Check sheet for the modelled part. Datum: model origin and axes. Units: mm. A direction names the side the tool comes from. Give positions to 0.01 mm unless a question says otherwise; leave off trailing zeros. Write each loop counter-clockwise with the first axis right and the second up, starting at its lowest first coordinate (ties: lowest second). Pieces come first, ordered by that corner, then holes. Notation, with made-up numbers: M -11.75,-35 L 6.25,-35 A28 ccw 6.25,4 Z; hole C 66,55 d1. An arc over 180 degrees is marked long. Write item = value, one per line. Start each with the question number.
1) Cross-section at A-A, the plane x = 24.5. Record the cut outline in (y, z), plus the area to 3 significant figures.
2) Go/stop test with flat-tipped pins: pin 1 (8 mm diameter, centred on x = -19.5, y = 4, fed in from -Z); pin 2 (8.5 mm diameter, centred on x = 1.5, z = 253.5, fed in from +Y); pin 3 (4 mm diameter, centred on x = 11.5, y = 13.5, fed in from +Z). Record where each tip stops, or that it passes through.
3) Scan lines: line 1 along Z through (x, y) = (-3, 17.5); line 2 along Y through (x, z) = (-28.5, 328.5); line 3 along Z through (x, y) = (-11, 3.25). Record each from-to range of solid material in increasing order. Write a range as [from, to].
4) Mould release check, pull along X, two halves, no side actions. Record for faces 4 (the cylindrical face through (-3.9, 3.4, 198.1)), 5 (the flat face through (-31.75, 7, 95)), 6 (the flat face through (0, 0, 174)): released by +X, released by -X, zero draft, split by the parting line, or undercut.
5) Cross-section at B-B, the plane y = 14.5. Record the cut outline in (x, z), plus the area to 3 significant figures.
6) Access from +Z, -Z, +X, -X, +Y, -Y to the whole of each face (thin tool, end or side, straight path). Record for faces 1 (the flat face through (0, 12, 152.4)), 2 (the flat face through (2, 2.013, 204)), 3 (the flat face through (31.75, 7, 95)).
7) Cross-section at C-C, the plane z = 288. Record the cut outline in (x, y).
```python
from build123d import *

# Parameters (mm, degrees)
SKETCH1_W                       = 63.5
SKETCH1_H                       = 19.05
BOSS_EXTRUDE1_DEPTH             = 349.25
SKETCH3_W                       = 196.85
SKETCH3_H                       = 14.2875
CUT_EXTRUDE1_DEPTH              = 356.486589058
CUT_EXTRUDE2_DEPTH              = 356.486589058
CBORE_FOR_M5_SBHCS1_D           = 5.5
CBORE_FOR_M5_SBHCS1_CBORE_D     = 10.5
CBORE_FOR_M5_SBHCS1_CBORE_DEPTH = 2.75


with BuildPart() as part:
    # Sketch1 → Boss-Extrude1 (new body)
    with BuildSketch(Plane.XY):
        with Locations((0, 9.525)):
            Rectangle(SKETCH1_W, SKETCH1_H)
    extrude(amount=BOSS_EXTRUDE1_DEPTH)

    # Sketch3 → Cut-Extrude1 (cut, through all)
    with BuildSketch(Plane(origin=(31.75, 0, 0), x_dir=(0, 0, -1), z_dir=(1, 0, 0))):
        with Locations((-250.825, 11.90625)):
            Rectangle(SKETCH3_W, SKETCH3_H)
    extrude(amount=-CUT_EXTRUDE1_DEPTH, mode=Mode.SUBTRACT)

    # Sketch14 → Cut-Extrude2 (cut, through all)
    with BuildSketch(Plane(origin=(31.75, 0, 0), x_dir=(0, 0, -1), z_dir=(1, 0, 0))):
        Polygon((-3.863258779, 0), (0, 0), (0, 10.924113624), align=None)
    extrude(amount=-CUT_EXTRUDE2_DEPTH, mode=Mode.SUBTRACT)

    # CBORE for M5 SBHCS1 (through all)
    with Locations(Plane(origin=(0, 4.7625, 0), x_dir=(1, 0, 0), z_dir=(0, 1, 0))):
        with Locations((0, -201.6125), (0, -250.825), (0, -300.0375)):
            CounterBoreHole(CBORE_FOR_M5_SBHCS1_D / 2, CBORE_FOR_M5_SBHCS1_CBORE_D / 2, CBORE_FOR_M5_SBHCS1_CBORE_DEPTH)


solid = part.part
```
Reply:
q1.outline = M 0,3.86 L 10.92,0 L 19.05,0 L 19.05,152.4 L 4.76,152.4 L 4.76,349.25 L 0,349.25 Z
q1.area = 3,820 mm2
q2.pin_1 = 1.03
q2.pin_2 = 4.76
q2.pin_3 = 152.4
q3.line_1 = [0, 152.4]
q3.line_2 = [0, 4.76]
q3.line_3 = [2.71, 349.25]
q4.face_4 = undercut
q4.face_5 = released by -X
q4.face_6 = zero draft
q5.outline = M -31.75,0 L 31.75,0 L 31.75,152.4 L -31.75,152.4 Z
q5.area = 9,680 mm2
q6.face_1 = +Z, +X, -X, +Y
q6.face_2 = +Y
q6.face_3 = +Z, -Z, +X, +Y, -Y
q7.outline = M -31.75,0 L 31.75,0 L 31.75,4.76 L -31.75,4.76 Z
